```python
from build123d import *

# Parameters (mm, degrees)
F0_R      = 57.861
F1_DEPTH  = 253.413677
F1_FACE_R = 57.861
F2_DEPTH  = 144.836873
F5_DEPTH  = 25.4


with BuildPart() as f1:
    # F0 (on Front) → F1 (new body)
    with BuildSketch(Plane.XZ):
        with Locations((70.250988, 58.846217)):
            Circle(F0_R)
    extrude(amount=F1_DEPTH)

    # F1_face (on face) → F2 (join)
    with BuildSketch(Plane(origin=(70.250988, -253.413677, 58.846217), x_dir=(1, 0, 0), z_dir=(0, -1, 0))):
        Circle(F1_FACE_R)
    extrude(amount=F2_DEPTH)

    # F4 (on face) → F5 (join)
    with BuildSketch(Plane.XZ.offset(398.25055)):
        with BuildLine():
            add(Edge.make_bspline(
                [(69.40268, 33.042915), (96.414929, 10.176068), (112.361828, 56.401889), (128.308728, 102.62771), (85.34958, 79.268736), (42.390431, 55.909762), (69.40268, 33.042915)],
                knots=[0, 0, 0, 2.094395, 2.094395, 4.18879, 4.18879, 6.283185, 6.283185, 6.283185], degree=2, weights=[1, 0.5, 1, 0.5, 1, 0.5, 1]))
        make_face()
    extrude(amount=F5_DEPTH)


solid = f1.part
```
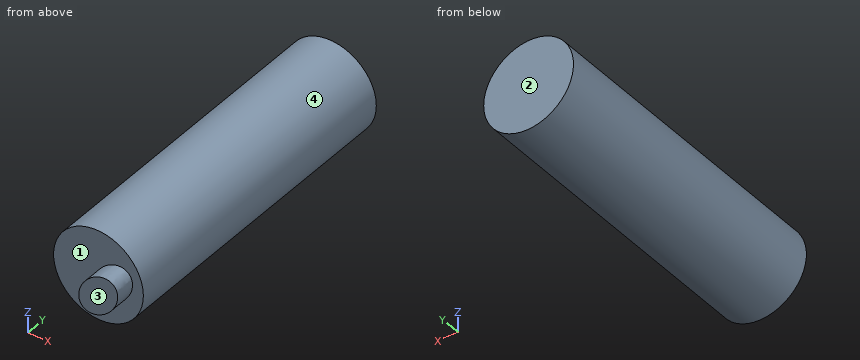
Source: CAD feature listing. Evaluate the final solid. Frame: model axes, mm. Face numbers are marked on the shaded views. A direction names the side the tool comes from. Give positions to 0.01 mm unless a question says otherwise; leave off trailing zeros. Loops run counter-clockwise (first coordinate to the right, second up) from the corner with the lowest first, then second, coordinate; pieces in that order, holes last. Notation, with made-up numbers: (31, 14.25) -> (42, 14.25) arc R16 ccw to (42, 26.25) -> close; hole circle Ø10 at (-3, 76). An arc over 180 degrees is marked (long way). Use a Markdown table: item, result. Add a question column.
(1) Access query for the marked faces 1 and 2. Directions: +Z, -Z, +X, -X, +Y, -Y. A direction counts if a zero-diameter tool reaches every point of the face in a straight line with its end or side. Return the directions, or none.
(2) Section query A-A (x = 28.5). Output: boundary loops of the cut face in (y, z).
(3) Ray query, line 1 (Y direction, x = 119, z = 72.5); line 2 (Z direction, x = 45, y = -138); line 3 (Z direction, x = 24.5, y = -316.5). Return the intervals inside material, ascending.
(4) Section query B-B (z = 8). Output: boundary loops of the cut face in (x, y).
(5) First-contact query: pin 1 Ø12 at (x, z) = (44.5, 58.5) entering from -Y; pin 2 Ø8 at (x, y) = (67.5, -118.5) entering from -Z; pin 3 Ø4 at (y, z) = (-163.5, 22) entering from +X. Flat tips, straight axial feed; report the tip coordinate or a pass-through.
(6) Pull-direction query (Z, two-part tool) for the marked faces 3 and 4; classes: +Z half, -Z half, draft (parallel to the pull), parting line (faces both ways), or undercut.
(7) Section query C-C (y = -374.5). Output: boundary loops of the cut face in (x, z).
Checked values:
| question | item | result |
|---|---|---|
| 1 | face 1 | -Y |
| 1 | face 2 | +Z, -Z, +X, -X, +Y |
| 2 | outline | (-398.25, 18.79) -> (0, 18.79) -> (0, 98.91) -> (-398.25, 98.91) -> close |
| 3 | line 1 | -398.25 to 0 |
| 3 | line 2 | 6.79 to 110.91 |
| 3 | line 3 | 23.42 to 94.27 |
| 4 | outline | (42.64, -398.25) -> (97.87, -398.25) -> (97.87, 0) -> (42.64, 0) -> close |
| 5 | pin 1 | y = -398.25 |
| 5 | pin 2 | z = 0.99 |
| 5 | pin 3 | x = 116.44 |
| 6 | face 3 | draft |
| 6 | face 4 | parting line |
| 7 | outline | circle Ø115.72 at (70.25, 58.85) |
